Source: CAD feature listing. Evaluate the final solid. Frame: model axes, mm. Give positions to 0.01 mm unless a question says otherwise; leave off trailing zeros. Loops run counter-clockwise (first coordinate to the right, second up) from the corner with the lowest first, then second, coordinate; pieces in that order, holes last.
```python
from build123d import *

# Parameters (mm, degrees)
SKETCH_W             = 38
SKETCH_H             = 36
PAD_DEPTH            = 23
POCKET_DEPTH         = 38.001
POCKET001_DEPTH      = 18.001
POCKET001_DEPTH_BACK = -18.001


with BuildPart() as part:
    # Sketch → Pad (new body)
    with BuildSketch(Plane.XY):
        Rectangle(SKETCH_W, SKETCH_H)
    extrude(amount=PAD_DEPTH)

    # Sketch001 (on Face2 of Pad) → Pocket (cut, through all)
    with BuildSketch(Plane.YZ.offset(19)):
        Polygon((-18, 4), (-21, 4), (-21, 26), (21, 26), (21, 4), (18, 4), (18, 23), (16.3, 23), (16.3, 4), (13.1, 4), (13.1, 23), (11.4, 23), (11.4, 4), (8.2, 4), (8.2, 23), (6.5, 23), (6.5, 4), (3.3, 4), (3.3, 23), (1.6, 23), (1.6, 7), (0.9, 7), (0.9, 4), (-0.9, 4), (-0.9, 7), (-1.6, 7), (-1.6, 23), (-3.3, 23), (-3.3, 4), (-6.5, 4), (-6.5, 23), (-8.2, 23), (-8.2, 4), (-11.4, 4), (-11.4, 23), (-13.1, 23), (-13.1, 4), (-16.3, 4), (-16.3, 23), (-18, 23), align=None)
    extrude(amount=-POCKET_DEPTH, mode=Mode.SUBTRACT)

    # Sketch002 → Pocket001 (cut, two sides)
    with BuildSketch(Plane.XZ) as pocket001_sk:
        Polygon((-19, 23), (-19, 4), (-22.4, 4), (-22.4, 26.4), (22.4, 26.4), (22.4, 4), (19, 4), (19, 23), (15.5, 23), (15.5, 4), (12.1, 4), (12.1, 23), (8.6, 23), (8.6, 4), (5.2, 4), (5.2, 23), (1.7, 23), (1.7, 4), (-1.7, 4), (-1.7, 23), (-5.2, 23), (-5.2, 4), (-8.6, 4), (-8.6, 23), (-12.1, 23), (-12.1, 4), (-15.5, 4), (-15.5, 23), align=None)
    extrude(amount=-POCKET001_DEPTH, mode=Mode.SUBTRACT)
    extrude(pocket001_sk.sketch, amount=-POCKET001_DEPTH_BACK, mode=Mode.SUBTRACT)


solid = part.part
```
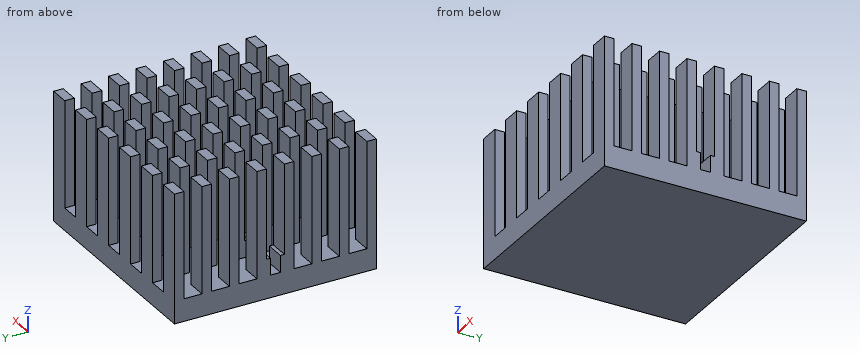
(1) First-contact query: pin 1 (2 mm diameter, centred on x = -4, y = -9.5, fed in from +Z). Flat tip, straight axial feed; report the tip coordinate or a pass-through.
A:
pin 1: stops at z = 4
(2) Section A-A, the plane y = 7. Return the cut outline in (x, z), then the cut area to 3 significant figures.
A:
outline: (-19, 0) - (19, 0) - (19, 23) - (15.5, 23) - (15.5, 4) - (12.1, 4) - (12.1, 23) - (8.6, 23) - (8.6, 4) - (5.2, 4) - (5.2, 23) - (1.7, 23) - (1.7, 4) - (-1.7, 4) - (-1.7, 23) - (-5.2, 23) - (-5.2, 4) - (-8.6, 4) - (-8.6, 23) - (-12.1, 23) - (-12.1, 4) - (-15.5, 4) - (-15.5, 23) - (-19, 23) - close
area: 551 mm2
(3) Ray query, line 1 along X through (y, z) = (-12, 18.5); line 2 along Z through (x, y) = (13, -11); line 3 along Z through (x, y) = (9, 1.5). Return the intervals inside material, ascending.
A:
line 1: x = -19 to -15.5, -12.1 to -8.6, -5.2 to -1.7, 1.7 to 5.2, 8.6 to 12.1, 15.5 to 19
line 2: z = 0 to 4
line 3: z = 0 to 7
(4) Section B-B, the plane z = 17. Count the separate pieces of the cut face and the enclosed holes in it, then the cut area to 3 significant figures.
A:
separate pieces: 48
enclosed holes: 0
area: 286 mm2
(5) Section C-C, the plane x = 7.5. Return the cut outline in (y, z).
A:
outline: (-18, 0) - (18, 0) - (18, 4) - (-18, 4) - close
